Geometry check sheet. Reference: the model listing, model coordinates, mm. A direction names the side the tool comes from. Give positions to 0.01 mm unless a question says otherwise; leave off trailing zeros. Write each loop counter-clockwise with the first axis right and the second up, starting at its lowest first coordinate (ties: lowest second). Pieces come first, ordered by that corner, then holes. Notation, with made-up numbers: M -31,-1.5 L 14,-1.5 A19 ccw 14,25.5 Z; hole C 22.5,-22 d5. An arc over 180 degrees is marked long. One line per item, written item: value. Start each with the question number.
1. Gauge pin test, flat ends, axial feed: pin 1 (1.5 mm diameter, centred on x = 3.5, y = -5, fed in from -Z); pin 2 (1.5 mm diameter, centred on x = -15.5, y = -15.5, fed in from +Z); pin 3 (3 mm diameter, centred on x = 15.5, y = 15.5, fed in from +Z); pin 4 (2 mm diameter, centred on x = 0.5, z = 52.5, fed in from +Y). Record the tip position at first contact, or that the pin passes through.
2. Cross-section at D-D on z = 45.5. Record the cut outline in (x, y).
3. Cross-section at A-A on x = 0. Record the cut outline in (y, z), then the cut area to 3 significant figures.
4. Cross-section at B-B on z = 17. Record the cut outline in (x, y).
5. Release check for a two-part mould opening along X. For faces 1 (the face through (-15.55, 15.29, 31.88)), 2 (the face through (21.15, 0, 20)), 3 (the face through (0, -21.15, 20)) record: pulls with the +X half, pulls with the -X half, needs draft (parallel to the pull), parting line crosses it, or undercut.
6. Scan lines: line 1 (Y direction, x = 15.5, z = 36); line 2 (Y direction, x = -14.5, z = 39.5). Record each from-to range of solid material in increasing order.
7. Cross-section at C-C on y = 13. Record the cut outline in (x, z).
8. Tool access check on faces 4 (the face through (-2.38, -10.74, 40.99)), 5 (the face through (-21.15, 0, 20)). Record the directions out of +Z, -Z, +X, -X, +Y, -Y that give a thin tool (end or side, any length) a straight path to the whole face; none if there is none.
from build123d import *

# Parameters (mm, degrees)
SKETCH_1_W             = 42.3
SKETCH_1_H             = 42.3
EXTRUDE_1_DEPTH        = 40
SKETCH_2_R             = 11
EXTRUDE_2_DEPTH        = 2
SKETCH_3_R             = 2.5
EXTRUDE_3_DEPTH        = 15
SKETCH_4_W             = 22.313934425
SKETCH_4_H             = 9.701954983
CUT_EXTRUDE_1_DEPTH    = 11
CHAMFER_1_SIZE         = 4
HOLE_WIZARD_M3_1_D     = 2.5
HOLE_WIZARD_M3_1_DEPTH = 7.5
HOLE_WIZARD_M3_1_TIP   = 0.751075774


with BuildPart() as part:
    # 草图1 → 凸台-拉伸1 (new body)
    with BuildSketch(Plane.XY):
        Rectangle(SKETCH_1_W, SKETCH_1_H)
    extrude(amount=EXTRUDE_1_DEPTH)

    # 草图2 → 凸台-拉伸2 (add)
    with BuildSketch(Plane.XY.offset(40)):
        Circle(SKETCH_2_R)
    extrude(amount=EXTRUDE_2_DEPTH)

    # 草图3 → 凸台-拉伸3 (add)
    with BuildSketch(Plane.XY.offset(42)):
        Circle(SKETCH_3_R)
    extrude(amount=EXTRUDE_3_DEPTH)

    # 草图4 → 切除-拉伸1 (cut, symmetric)
    with BuildSketch(Plane(origin=(0, 0, 0), x_dir=(0, 0, -1), z_dir=(1, 0, 0))):
        with Locations((-58.156967212, 6.350977492)):
            Rectangle(SKETCH_4_W, SKETCH_4_H)
    extrude(amount=CUT_EXTRUDE_1_DEPTH, both=True, mode=Mode.SUBTRACT)

    # 倒角1
    chamfer_1_edges = [part.edges().sort_by_distance(p)[0] for p in [
        (21.15, -21.15, 20),
        (-21.15, -21.15, 20),
        (-21.15, 21.15, 20),
        (21.15, 21.15, 20),
    ]]
    chamfer(chamfer_1_edges, length=CHAMFER_1_SIZE)

    # M3 螺纹孔1
    with Locations(Plane.XY.offset(40)):
        with Locations((-15.5, 15.5), (-15.5, -15.5), (15.5, -15.5), (15.5, 15.5)):
            Hole(HOLE_WIZARD_M3_1_D / 2, depth=HOLE_WIZARD_M3_1_DEPTH)
            with Locations((0, 0, -(HOLE_WIZARD_M3_1_DEPTH + HOLE_WIZARD_M3_1_TIP / 2))):  # 118° drill point
                Cone(0, HOLE_WIZARD_M3_1_D / 2, HOLE_WIZARD_M3_1_TIP, mode=Mode.SUBTRACT)


solid = part.part
Report:
1. pin 1: stops at z = 0
1. pin 2: stops at z = 32.2
1. pin 3: stops at z = 40
1. pin 4: stops at y = 1.5
2. outline: C 0,0 d5
3. outline: M -21.15,0 L 21.15,0 L 21.15,40 L 11,40 L 11,42 L 2.5,42 L 2.5,47 L 1.5,47 L 1.5,57 L -2.5,57 L -2.5,42 L -11,42 L -11,40 L -21.15,40 Z
3. area: 1,800 mm^2
4. outline: M -21.15,-17.15 L -17.15,-21.15 L 17.15,-21.15 L 21.15,-17.15 L 21.15,17.15 L 17.15,21.15 L -17.15,21.15 L -21.15,17.15 Z
5. face 1: undercut
5. face 2: pulls with the +X half
5. face 3: needs draft
6. line 1: y = -21.15 to -16.75, -14.25 to 14.25, 16.75 to 21.15
6. line 2: y = -21.15 to -16.25, -14.75 to 14.75, 16.25 to 21.15
7. outline: M -21.15,0 L 21.15,0 L 21.15,40 L -21.15,40 Z
8. face 4: +Z
8. face 5: +Z, -Z, -X, +Y, -Y
